For this review, use the dimensioned drawing (mm, ordinates from the lowest corner) and the shaded views. Give positions to 0.01 mm unless a question says otherwise; leave off trailing zeros. Write each loop counter-clockwise with the first axis right and the second up, starting at its lowest first coordinate (ties: lowest second). Pieces come first, ordered by that corner, then holes. Notation, with made-up numbers: (19, 84.5) -> (54, 84.5) arc R15 cw to (54, 103.5) -> close; hole circle Ø9 at (74.5, -13.5). An arc over 180 degrees is marked (long way). Return JSON: item names as keys, results as strings.
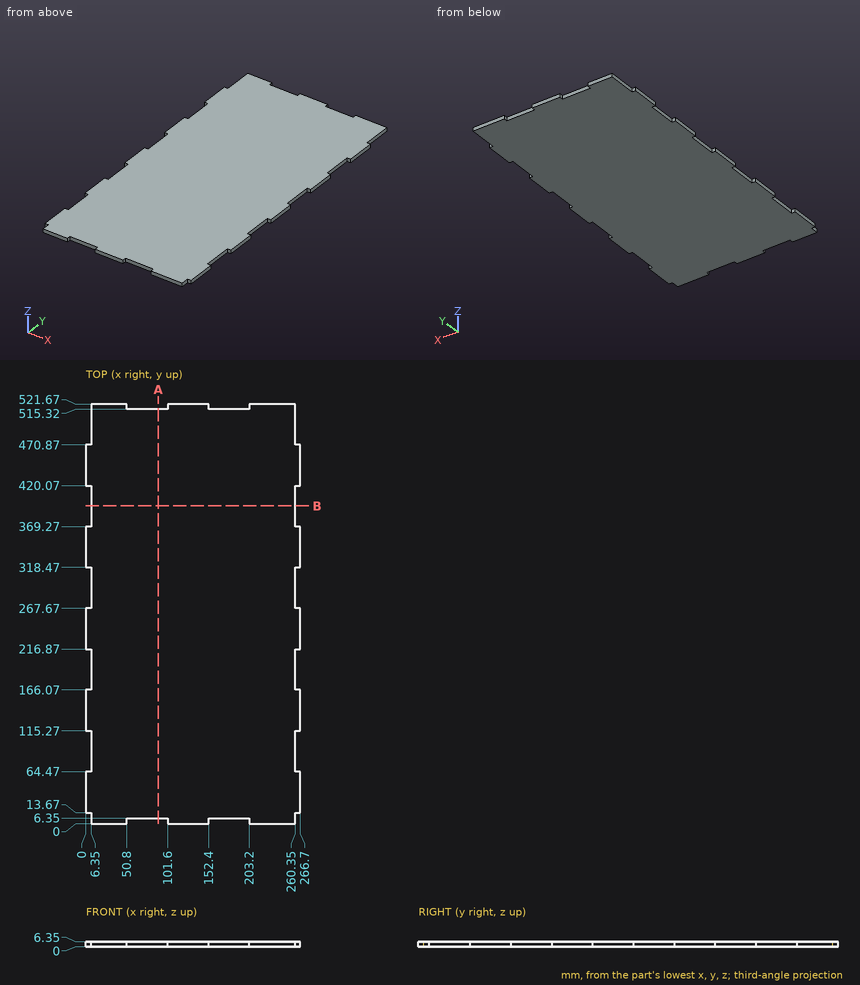
1. For pin 1 (1.9 mm diameter, centred on x = 2, z = 4, fed in from -Y); pin 2 (1.9 mm diameter, centred on x = 4, z = 2, fed in from +Y); pin 3 (1 mm diameter, centred on x = 68, z = 3, fed in from +Y), all flat-tipped, find the tip position at first contact; note any pin that passes through.
Results found:
{"pin 1": "stops at y = 13.67", "pin 2": "stops at y = 470.87", "pin 3": "stops at y = 515.32"}
2. Add section B-B, the plane y = 395. State the section outline as (x, z) points.
Results found:
{"outline": "(6.35, 0) -> (260.35, 0) -> (260.35, 6.35) -> (6.35, 6.35) -> close"}
3. Add section A-A, the plane x = 90. State the section outline as (y, z) points, plus the area to 3 significant figures.
Results found:
{"outline": "(6.35, 0) -> (515.32, 0) -> (515.32, 6.35) -> (6.35, 6.35) -> close", "area": "3,230 mm²"}
4. To check wall thickness, follow probe 1 along Y at (x, z) = (203, 5); probe 2 along X at (y, z) = (177, 4.5). State the ranges of each line that lie inside material, in increasing order.
Results found:
{"probe 1": "y = 6.35 to 515.32", "probe 2": "x = 6.35 to 260.35"}
